For this review, use the dimensioned drawing (mm, ordinates from the lowest corner) and the shaded views. A direction names the side the tool comes from. Coordinates: 2 decimals unless noted, no trailing zeros. Write each loop counter-clockwise with the first axis right and the second up, starting at its lowest first coordinate (ties: lowest second). Pieces come first, ordered by that corner, then holes.
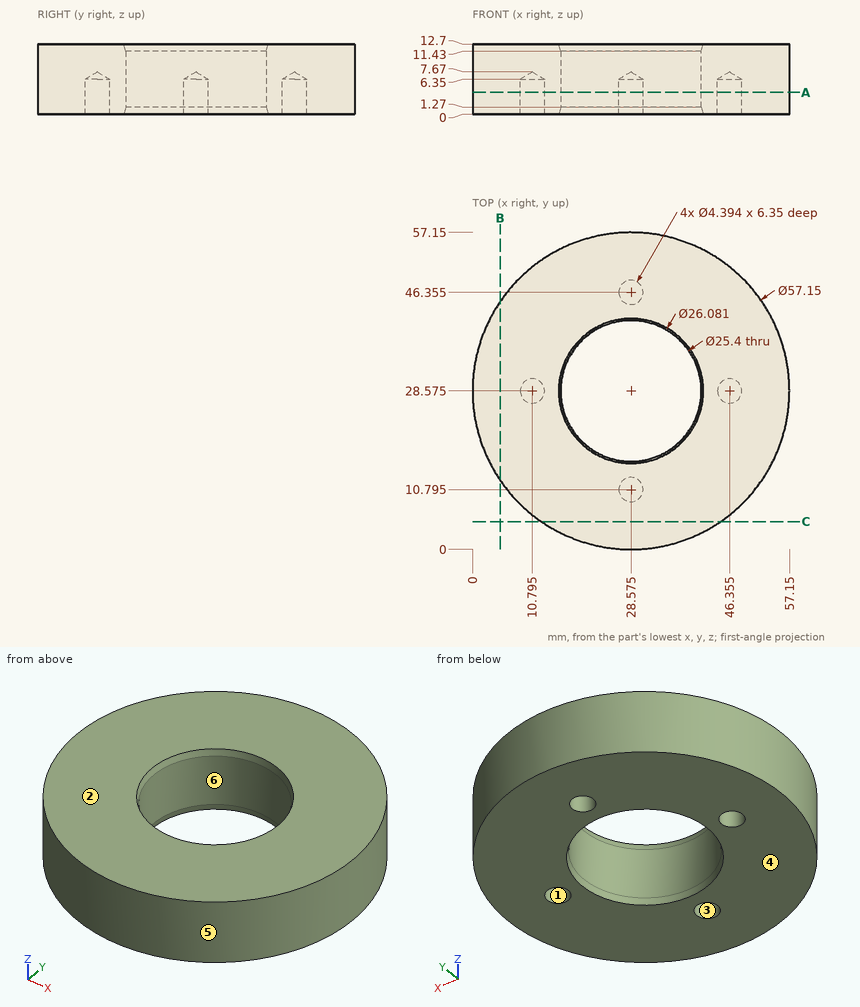
Item 1: Take a section at B-B, the plane x = 5. Write out the cut boundary in (y, z).
Solved:
outline: (12.43, 0) - (44.72, 0) - (44.72, 12.7) - (12.43, 12.7) - close
Item 2: Take a section at A-A, the plane z = 4. Count the separate pieces of the cut face and the enclosed holes in it, plus the area to 3 significant figures.
Solved:
separate pieces: 1
enclosed holes: 5
area: 2,000 mm2
Item 3: Mouldability with a two-part tool opening along Y and no side actions: class the marked faces 3, 4, 5 and 6 as pulls with the +Y half, pulls with the -Y half, needs draft (parallel to the pull), parting line crosses it, or undercut.
Solved:
face 3: undercut
face 4: needs draft
face 5: parting line crosses it
face 6: undercut
Item 4: For pin 1 (3.5 mm diameter, centred on x = 10.795, y = 28.575, fed in from -Z); pin 2 (15 mm diameter, centred on x = 28.575, y = 28.575, fed in from +Z); pin 3 (3 mm diameter, centred on x = 11, z = 4.5, fed in from -Y); pin 4 (3 mm diameter, centred on x = 30, z = 4, fed in from -Y), all flat-tipped, find the tip position at first contact; note any pin that passes through.
Solved:
pin 1: stops at z = 6.62
pin 2: passes through
pin 3: stops at y = 4.95
pin 4: stops at y = 0
Item 5: Machinability: for the marked faces 1 and 2, which of the approach directions +Z, -Z, +X, -X, +Y, -Y give a long, thin tool a straight path to every point of the face, cutting with its end or side? Answer none if there is none.
Solved:
face 1: -Z
face 2: +Z, +X, -X, +Y, -Y
Item 6: To check wall thickness, follow line 1 along X through (y, z) = (30, 1.5) (1 decimal); line 2 along Y through (x, z) = (27, 0.75) (1 decimal); line 3 along X through (y, z) = (22, 11) (1 decimal). State the ranges of each line that lie inside material, in increasing order.
Solved:
line 1: x = 0 to 9.1, 12.5 to 16, 41.2 to 44.7, 48 to 57.1
line 2: y = 0 to 9.3, 12.3 to 15.8, 41.3 to 44.8, 47.9 to 57.1
line 3: x = 0.8 to 17.7, 39.4 to 56.4
